Verification items for the finished model (mm, model axes). Give positions to 0.01 mm unless a question says otherwise; leave off trailing zeros.
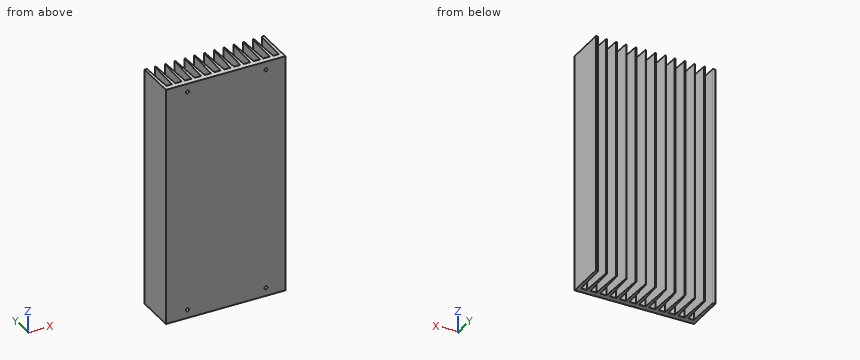
from build123d import *

# Parameters (mm, degrees)
EXTRUDE_1_DEPTH       = 245
EXTRUDE_3_DEPTH       = 245
PATTERN_CURVE_1_COUNT = 11
PATTERN_CURVE_1_PITCH = 10
SKETCH_3_R            = 1.6
CUT_EXTRUDE_1_DEPTH   = 6


with BuildPart() as part:
    # Эскиз1 → Вытянуть1 (new body)
    with BuildSketch(Plane.XY):
        with BuildLine():
            Line((0, 40), (1.528979332, 40))
            ThreePointArc((1.528979332, 40), (2.225614441, 39.717425624), (2.528547087, 39.029399052))
            Line((2.528547087, 39.029399052), (3.5, 6))
            Line((3.5, 6), (118.5, 6))
            Line((118.5, 6), (119.471452913, 39.029399052))
            ThreePointArc((119.471452913, 39.029399052), (119.774385559, 39.717425624), (120.471020668, 40))
            Line((120.471020668, 40), (122, 40))
            Line((122, 40), (122, 0))
            Line((122, 0), (0, 0))
            Line((0, 0), (0, 40))
        make_face()
    extrude(amount=EXTRUDE_1_DEPTH)

    # Эскиз2 → Вытянуть3 (add)
    with BuildSketch(Plane.XY.offset(245)):
        with BuildLine():
            Line((10.5, 39.5), (9.25, 6))
            Line((9.25, 6), (12.75, 6))
            Line((12.75, 6), (11.5, 39.5))
            ThreePointArc((11.5, 39.5), (11, 40), (10.5, 39.5))
        make_face()
    extrude_3 = extrude(amount=-EXTRUDE_3_DEPTH)

    # Кривая1: Вытянуть3 ×11
    with Locations(*[(i * PATTERN_CURVE_1_PITCH, 0, 0) for i in range(1, PATTERN_CURVE_1_COUNT)]):
        add(extrude_3)

    # Эскиз3 → Вырез-Вытянуть1 (cut)
    with BuildSketch(Plane.XZ):
        with Locations((22, 236.5)):
            Circle(SKETCH_3_R)
        with Locations((102, 236.5)):
            Circle(SKETCH_3_R)
        with Locations(Location((102, 8.5, 0), (0, 0, 62.046813117))):
            Circle(SKETCH_3_R)
        with Locations(Location((22, 8.5, 0), (0, 0, 62.046813117))):
            Circle(SKETCH_3_R)
    extrude(amount=-CUT_EXTRUDE_1_DEPTH, mode=Mode.SUBTRACT)


solid = part.part
Item 1: Scan lines: line 1 along Z through (x, y) = (22, 3); line 2 along X through (y, z) = (1.95, 8.5); line 3 along Y through (x, z) = (27.5, 210). Record each from-to range of solid material in increasing order.
Answer key:
line 1: z = 0 to 6.9, 10.1 to 234.9, 238.1 to 245
line 2: x = 0 to 20.4, 23.6 to 100.4, 103.6 to 122
line 3: y = 0 to 6
Item 2: Depth check by flat-ended pin: pin 1 (2.5 mm diameter, centred on x = 21, z = 8.5, fed in from -Y); pin 2 (2 mm diameter, centred on x = 85, z = 103, fed in from +Y). Enter the tip coordinate at first touch or a pass-through.
Answer key:
pin 1: stops at y = 0
pin 2: stops at y = 6
Item 3: Sectioned sample at A-A on y = 30. State how many separate pieces and enclosed holes the cut face has, then the cut area to 3 significant figures.
Answer key:
separate pieces: 13
enclosed holes: 0
area: 5,970 mm2
